Verification items for the finished model (mm, model axes). Face numbers are marked on the shaded views. A direction names the side the tool comes from. Coordinates: 2 decimals unless noted, no trailing zeros. Write each loop counter-clockwise with the first axis right and the second up, starting at its lowest first coordinate (ties: lowest second). Pieces come first, ordered by that corner, then holes.
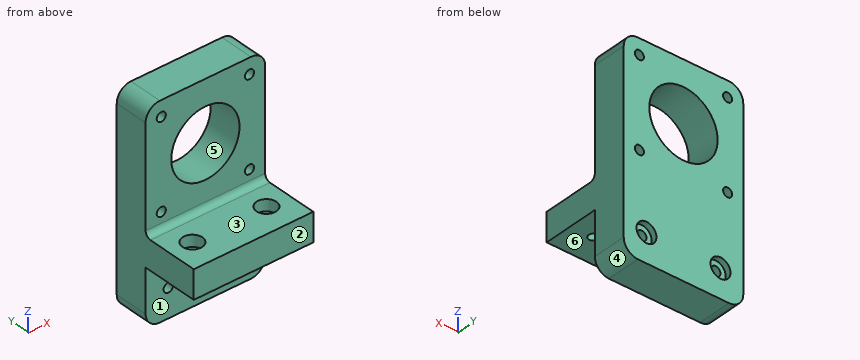
```python
from build123d import *

# Parameters (mm, degrees)
F0_W     = 42
F0_H     = 10
F1_DEPTH = 20
F0_H_2   = 42
F0_R     = 1.6
F0_R_2   = 12
F0_H_3   = 20.2
F0_R_3   = 3.5
F0_H_4   = 0.1999993771
F2_DEPTH = 12
F3_R     = 1.7
F4_DEPTH = 25
F3_R_2   = 3.5
F5_DEPTH = 4
F0_R_4   = 1.7
F6_DEPTH = 12
F7_R     = 3.5
F7_R_2   = 1.7
F8_DEPTH = 2
F9_R     = 5
F10_R    = 2


# Not quite as in the source:
# - a feature names something its author has since deleted; it is built from what else it names


with BuildPart() as f1:
    # F0 (on Front) → F1 (new body)
    with BuildSketch(Plane.XZ):
        with Locations((0, -26.1999993771)):
            Rectangle(F0_W, F0_H)
    extrude(amount=F1_DEPTH)

    # F0 (on Front) → F2 (join)
    with BuildSketch(Plane.XZ):
        Rectangle(F0_W, F0_H_2)
        with Locations((-15.5, -15.5)):
            Circle(F0_R, mode=Mode.SUBTRACT)
        with Locations((15.5, -15.5)):
            Circle(F0_R, mode=Mode.SUBTRACT)
        with Locations((-15.5, 15.5)):
            Circle(F0_R, mode=Mode.SUBTRACT)
        Circle(F0_R_2, mode=Mode.SUBTRACT)
        with Locations((15.5, 15.5)):
            Circle(F0_R, mode=Mode.SUBTRACT)
        with Locations((0, -26.1999993771)):
            Rectangle(F0_W, F0_H)
        with Locations((0, -41.2999993771)):
            Rectangle(F0_W, F0_H_3)
        with Locations((-13, -41.2999993771)):
            Circle(F0_R_3, mode=Mode.SUBTRACT)
        with Locations((13, -41.2999993771)):
            Circle(F0_R_3, mode=Mode.SUBTRACT)
        with Locations((0, -21.0999996886)):
            Rectangle(F0_W, F0_H_4)
    extrude(amount=-F2_DEPTH)

    # F3 (on face) → F4 (cut)
    with BuildSketch(Plane.XY.offset(-21.1999993771)):
        with Locations((-13, -10)):
            Circle(F3_R)
        with Locations((13, -10)):
            Circle(F3_R)
    extrude(amount=-F4_DEPTH, mode=Mode.SUBTRACT)

    # F3 (on face) → F5 (cut)
    with BuildSketch(Plane.XY.offset(-21.1999993771)):
        with Locations((-13, -10)):
            Circle(F3_R_2)
        with Locations((-13, -10)):
            Circle(F3_R, mode=Mode.SUBTRACT)
        with Locations((13, -10)):
            Circle(F3_R_2)
        with Locations((13, -10)):
            Circle(F3_R, mode=Mode.SUBTRACT)
    extrude(amount=-F5_DEPTH, mode=Mode.SUBTRACT)

    # F0 (on Front) → F6 (join)
    with BuildSketch(Plane.XZ):
        with Locations((13, -41.2999993771)):
            Circle(F0_R_3)
        with Locations((13, -41.2999993771)):
            Circle(F0_R_4, mode=Mode.SUBTRACT)
        with Locations((-13, -41.2999993771)):
            Circle(F0_R_3)
        with Locations((-13, -41.2999993771)):
            Circle(F0_R_4, mode=Mode.SUBTRACT)
    extrude(amount=-F6_DEPTH)

    # F7 (on face) → F8 (cut)
    with BuildSketch(Plane(origin=(0, 12, 0), x_dir=(-1, 0, 0), z_dir=(0, 1, 0))):
        with Locations((-13, -41.2999993771)):
            Circle(F7_R)
        with Locations((-13, -41.2999993771)):
            Circle(F7_R_2, mode=Mode.SUBTRACT)
        with Locations((13, -41.2999993771)):
            Circle(F7_R)
        with Locations((13, -41.2999993771)):
            Circle(F7_R_2, mode=Mode.SUBTRACT)
    extrude(amount=-F8_DEPTH, mode=Mode.SUBTRACT)

    # F9
    f9_edges = [f1.edges().sort_by_distance(p)[0] for p in [
        (21, 6, 21),
        (-21, 6, 21),
        (-21, 6, -51.399999),
        (21, 6, -51.399999),
    ]]
    fillet(f9_edges, radius=F9_R)

    # F10
    f10_edges = [f1.edges().sort_by_distance(p)[0] for p in [
        (0, 0, -21.199999),
    ]]
    fillet(f10_edges, radius=F10_R)


solid = f1.part
```
1. Tool access check on the marked faces 1, 2 and 3. Record the directions out of +Z, -Z, +X, -X, +Y, -Y that give a thin tool (end or side, any length) a straight path to the whole face; none if there is none.
2. Draft check along X on the marked faces 4, 5 and 6. Enter one of: pulls with the +X half, pulls with the -X half, needs draft (parallel to the pull), parting line crosses it, or undercut.
3. Sectioned sample at A-A, the plane z = -41.3. Record the boundary of the cut face in (x, y), and give its area (3 significant figures).
4. Sectioned sample at B-B, the plane z = 0. Record the boundary of the cut face in (x, y).
5. Sectioned sample at D-D, the plane x = 6. Record the boundary of the cut face in (y, z).
6. Gauge pin test, flat ends, axial feed: P1, Ø4, axis at x = 4, y = -16.5, coming from the +Z side; P2, Ø2.5, axis at x = 15.5, z = 15.5, coming from the +Y side; P3, Ø2, axis at x = -11.5, z = -40.5, coming from the +Y side; P4, Ø2, axis at x = -15.5, y = -2, coming from the +Z side. Record the tip position at first contact, or that the pin passes through.
7. Sectioned sample at C-C, the plane y = 2.5. Record the boundary of the cut face in (x, z), and give its area (3 significant figures).
8. Material ranges on L1, parallel to X at y = 11, z = -41; L2, parallel to Z at x = 13, y = 7; L3, parallel to Z at x = -6, y = -14.5, recorded low to high.
Outcome:
1. face 1: -Z, +X, -X, -Y
1. face 2: +Z, -Z, +X, -X, -Y
1. face 3: +Z, +X, -X, -Y
2. face 4: pulls with the +X half
2. face 5: undercut
2. face 6: needs draft
3. outline: (-21, 0) - (-14.7, 0) - (-14.7, 10) - (-16.5, 10) - (-16.5, 12) - (-21, 12) - close; (-11.3, 0) - (11.3, 0) - (11.3, 10) - (9.5, 10) - (9.5, 12) - (-9.5, 12) - (-9.5, 10) - (-11.3, 10) - close; (14.7, 0) - (21, 0) - (21, 12) - (16.5, 12) - (16.5, 10) - (14.7, 10) - close
3. area: 408 mm2
4. outline: (-21, 0) - (-12, 0) - (-12, 12) - (-21, 12) - close; (12, 0) - (21, 0) - (21, 12) - (12, 12) - close
5. outline: (-20, -31.2) - (0, -31.2) - (0, -51.4) - (12, -51.4) - (12, -10.39) - (0, -10.39) - (0, -19.2) arc R2 cw to (-2, -21.2) - (-20, -21.2) - close; (0, 10.39) - (12, 10.39) - (12, 21) - (0, 21) - close
6. P1: stops at z = -21.2
6. P2: passes through
6. P3: stops at y = 10
6. P4: stops at z = -20.93
7. outline: (-21, -46.4) arc R5 ccw to (-16, -51.4) - (16, -51.4) arc R5 ccw to (21, -46.4) - (21, 16) arc R5 ccw to (16, 21) - (-16, 21) arc R5 ccw to (-21, 16) - close; hole circle Ø3.2 at (-15.5, -15.5); hole circle Ø3.2 at (-15.5, 15.5); hole circle Ø3.4 at (-13, -41.3); hole circle Ø24 at (0, 0); hole circle Ø3.4 at (13, -41.3); hole circle Ø3.2 at (15.5, -15.5); hole circle Ø3.2 at (15.5, 15.5)
7. area: 2,520 mm2
8. L1: x = -21 to -16.49, -9.51 to 9.51, 16.49 to 21
8. L2: z = -51.4 to -43, -39.6 to 21
8. L3: z = -31.2 to -21.2
